Verification items for the finished model (mm, model axes). A direction names the side the tool comes from. Give positions to 0.01 mm unless a question says otherwise; leave off trailing zeros. Loops run counter-clockwise (first coordinate to the right, second up) from the corner with the lowest first, then second, coordinate; pieces in that order, holes last. Notation, with made-up numbers: (-7, 77) - (14, 77) arc R22 cw to (14, 110) - close; hole circle Ø6 at (52, -29.5). An arc over 180 degrees is marked (long way). One line per question, with ' | ' between items. Start each with the question number.
1. Section check A-A, the plane y = 16. Enter the section's corners in (x, z).
2. Section check C-C, the plane y = 3.5. Enter the section's corners in (x, z).
3. Thickness scan on line 1 along X through (y, z) = (16, 15.6); line 2 along Y through (x, z) = (19.75, 14.95); line 3 along X through (y, z) = (-17, 13.25). Record the ranges inside material, lowest first. Write a range as from..to.
4. Section check B-B, the plane z = 10.5. Enter the section's corners in (x, y).
5. Depth check by flat-ended pin: pin 1 Ø3 at (x, z) = (18.5, 8.5) entering from -Y; pin 2 Ø16 at (x, y) = (4, 4.5) entering from +Z; pin 3 Ø5.5 at (y, z) = (-15, 6.5) entering from -X. Enter the tip coordinate at first touch or a pass-through.
6. Mould release check, pull along Y, two halves, no side actions. Record for faces 1 (the face through (-16, 0, 1)), 2 (the face through (-16.792, -18.746, 3.522)), 3 (the face through (-17.4, 19.1, 1.4)): +Y half, -Y half, draft (parallel to the pull), parting line (faces both ways), or undercut.
7. Tool access check on faces 4 (the face through (-17.2, 12.7, 1.8)), 5 (the face through (17, 18.5, 12)), 6 (the face through (-17, -18.5, 12)), 7 (the face through (16, 0, 1)). Record the directions out of +Z, -Z, +X, -X, +Y, -Y that give a thin tool (end or side, any length) a straight path to the whole face; none if there is none.
8. Section check D-D, the plane x = 2.5. Enter the section's corners in (y, z), then the cut area to 3 significant figures.
from build123d import *

# Parameters (mm, degrees)
SKETCH1_W               = 32
SKETCH1_H               = 40
BOSS_EXTRUDE1_DEPTH     = 1.5
SKETCH2_R               = 1.2
BOSS_EXTRUDE2_DEPTH     = 16.5
CUT_EXTRUDE1_DEPTH      = 35.165955277
CUT_EXTRUDE1_DEPTH_BACK = 35.165955277
SKETCH4_W               = 10
SKETCH4_H               = 14.5
CHAMFER1_SIZE           = 2
FILLET1_R               = 5


with BuildPart() as part:
    # Sketch1 → Boss-Extrude1 (new body)
    with BuildSketch(Plane.XY):
        Rectangle(SKETCH1_W, SKETCH1_H)
    extrude(amount=BOSS_EXTRUDE1_DEPTH)

    # Sketch2 → Boss-Extrude2 (add)
    # profile 1 of 4: a face of its own
    with BuildSketch(Plane.XY):
        with BuildLine():
            Line((-16, 18.5), (-19.75, 18.5))
            ThreePointArc((-19.75, 18.5), (-22.25, 16), (-19.75, 13.5))
            Line((-19.75, 13.5), (-16, 13.5))
            Line((-16, 13.5), (-16, 18.5))
        make_face()
        with Locations((-19.75, 16)):
            Circle(SKETCH2_R, mode=Mode.SUBTRACT)
    # profile 2 of 4: a face of its own
    with BuildSketch(Plane.XY):
        with BuildLine():
            Line((16, 18.5), (16, 13.5))
            Line((16, 13.5), (19.75, 13.5))
            ThreePointArc((19.75, 13.5), (22.25, 16), (19.75, 18.5))
            Line((19.75, 18.5), (16, 18.5))
        make_face()
        with Locations(Location((19.75, 16, 0), (0, 0, 180))):
            Circle(SKETCH2_R, mode=Mode.SUBTRACT)
    # profile 3 of 4: a face of its own
    with BuildSketch(Plane.XY):
        with BuildLine():
            Line((16, -18.5), (19.75, -18.5))
            ThreePointArc((19.75, -18.5), (22.25, -16), (19.75, -13.5))
            Line((19.75, -13.5), (16, -13.5))
            Line((16, -13.5), (16, -18.5))
        make_face()
        with Locations((19.75, -16)):
            Circle(SKETCH2_R, mode=Mode.SUBTRACT)
    # profile 4 of 4: a face of its own
    with BuildSketch(Plane.XY):
        with BuildLine():
            Line((-16, -18.5), (-16, -13.5))
            Line((-16, -13.5), (-19.75, -13.5))
            ThreePointArc((-19.75, -13.5), (-22.25, -16), (-19.75, -18.5))
            Line((-19.75, -18.5), (-16, -18.5))
        make_face()
        with Locations(Location((-19.75, -16, 0), (0, 0, 180))):
            Circle(SKETCH2_R, mode=Mode.SUBTRACT)
    extrude(amount=BOSS_EXTRUDE2_DEPTH)

    # Sketch4 → Cut-Extrude1 (cut, two sides: drawn at the far end of the back side and taken through both)
    with BuildSketch(Plane(origin=(0, 0, 0), x_dir=(1, 0, 0), z_dir=(0, 1, 0)).offset(-CUT_EXTRUDE1_DEPTH_BACK)):
        with Locations((-23, -7.25)):
            Rectangle(SKETCH4_W, SKETCH4_H)
        with Locations((23, -7.25)):
            Rectangle(SKETCH4_W, SKETCH4_H)
    extrude(amount=CUT_EXTRUDE1_DEPTH + CUT_EXTRUDE1_DEPTH_BACK, mode=Mode.SUBTRACT)

    # Chamfer1
    # the kernel refuses this chamfer: 2 mm, written as the material it adds along each edge
    with BuildSketch(Plane(origin=(-16, -13.5, 0), x_dir=(-1, 0, 0), z_dir=(0, 0, 1)), Plane(origin=(-16, 13.5, 0), x_dir=(0, -1, 0), z_dir=(0, 0, 1)), Plane(origin=(16, -13.5, 0), x_dir=(0, 1, 0), z_dir=(0, 0, 1)), Plane(origin=(16, 13.5, 0), x_dir=(1, 0, 0), z_dir=(0, 0, 1))) as chamfer1_piece_1:
        Polygon((CHAMFER1_SIZE, 0), (0, -CHAMFER1_SIZE), (0, 0), align=None)
    extrude(amount=1.5)
    with BuildSketch(Plane(origin=(-16, -18.5, 0), x_dir=(0, -1, 0), z_dir=(0, 0, 1))) as chamfer1_piece_2_section:
        Polygon((CHAMFER1_SIZE, 0), (0, -CHAMFER1_SIZE), (0, 0), align=None)
    chamfer1_piece_2 = extrude(amount=1.5, mode=Mode.PRIVATE)
    chamfer1_piece_2 = split(chamfer1_piece_2, bisect_by=Plane(origin=(-16, -20, 0), z_dir=(0, 1, 0)), keep=Keep.TOP, mode=Mode.PRIVATE)
    add(chamfer1_piece_2)
    with BuildSketch(Plane(origin=(-16, 18.5, 0), x_dir=(0, 1, 0), z_dir=(0, 0, 1))) as chamfer1_piece_3_section:
        Polygon((CHAMFER1_SIZE, 0), (0, CHAMFER1_SIZE), (0, 0), align=None)
    chamfer1_piece_3 = extrude(amount=1.5, mode=Mode.PRIVATE)
    chamfer1_piece_3 = split(chamfer1_piece_3, bisect_by=Plane(origin=(-16, 20, 0), z_dir=(0, -1, 0)), keep=Keep.TOP, mode=Mode.PRIVATE)
    add(chamfer1_piece_3)
    with BuildSketch(Plane(origin=(16, -18.5, 0), x_dir=(1, 0, 0), z_dir=(0, 0, 1))) as chamfer1_piece_4_section:
        Polygon((CHAMFER1_SIZE, 0), (0, -CHAMFER1_SIZE), (0, 0), align=None)
    chamfer1_piece_4 = extrude(amount=1.5, mode=Mode.PRIVATE)
    chamfer1_piece_4 = split(chamfer1_piece_4, bisect_by=Plane(origin=(16, -20, 0), z_dir=(0, 1, 0)), keep=Keep.TOP, mode=Mode.PRIVATE)
    add(chamfer1_piece_4)
    with BuildSketch(Plane(origin=(16, 18.5, 0), x_dir=(0, 1, 0), z_dir=(0, 0, 1))) as chamfer1_piece_5_section:
        Polygon((CHAMFER1_SIZE, 0), (0, -CHAMFER1_SIZE), (0, 0), align=None)
    chamfer1_piece_5 = extrude(amount=1.5, mode=Mode.PRIVATE)
    chamfer1_piece_5 = split(chamfer1_piece_5, bisect_by=Plane(origin=(16, 20, 0), z_dir=(0, -1, 0)), keep=Keep.TOP, mode=Mode.PRIVATE)
    add(chamfer1_piece_5)

    # Fillet1
    # the kernel refuses this fillet: 5 mm, written as the material it adds along each edge
    with BuildSketch(Plane(origin=(-16, -13.5, 1.5), x_dir=(0, 0, 1), z_dir=(-1, 0, 0))) as fillet1_piece_1_section:
        with BuildLine():
            CenterArc((FILLET1_R, FILLET1_R), FILLET1_R, 180, 90)
            Line((0, FILLET1_R), (0, 0))
            Line((0, 0), (FILLET1_R, 0))
        make_face()
    fillet1_piece_1 = extrude(amount=14.5, mode=Mode.PRIVATE)
    fillet1_piece_1 = split(fillet1_piece_1, bisect_by=Plane(origin=(-17, -12.5, 1.5), z_dir=(0.7071067811865476, -0.7071067811865476, 0)), keep=Keep.TOP, mode=Mode.PRIVATE)
    add(fillet1_piece_1)
    with BuildSketch(Plane(origin=(-26.926785536, -18.5, 1.5), x_dir=(0, 0, 1), z_dir=(1, 0, 0))) as fillet1_piece_2_section:
        with BuildLine():
            CenterArc((3.570714214, 5), FILLET1_R, 224.427004001, 45.572995999)
            Line((0, 1.5), (0, 0))
            Line((0, 0), (3.570714214, 0))
        make_face()
    fillet1_piece_2 = extrude(amount=10.926785536, mode=Mode.PRIVATE)
    fillet1_piece_2 = split(fillet1_piece_2, bisect_by=Plane(origin=(-22.463392768, -14.036607232, 1.5), z_dir=(0.7071067811865476, 0.7071067811865476, 0)), keep=Keep.TOP, mode=Mode.PRIVATE)
    add(fillet1_piece_2)
    with BuildSketch(Plane(origin=(-30.5, 13.5, 1.5), x_dir=(0, 0, 1), z_dir=(1, 0, 0))) as fillet1_piece_3_section:
        with BuildLine():
            CenterArc((FILLET1_R, FILLET1_R), FILLET1_R, 180, 90)
            Line((0, FILLET1_R), (0, 0))
            Line((0, 0), (FILLET1_R, 0))
        make_face()
    fillet1_piece_3 = extrude(amount=14.5, mode=Mode.PRIVATE)
    fillet1_piece_3 = split(fillet1_piece_3, bisect_by=Plane(origin=(-24.25, 19.75, 1.5), z_dir=(0.7071067811865476, 0.7071067811865476, 0)), keep=Keep.TOP, mode=Mode.PRIVATE)
    add(fillet1_piece_3)
    with BuildSketch(Plane(origin=(-26.926785536, 18.5, 1.5), x_dir=(0, 0, 1), z_dir=(1, 0, 0))) as fillet1_piece_4_section:
        with BuildLine():
            CenterArc((3.570714214, -5), FILLET1_R, 90, 45.572995999)
            Line((0, -1.5), (0, 0))
            Line((0, 0), (3.570714214, 0))
        make_face()
    fillet1_piece_4 = extrude(amount=10.926785536, mode=Mode.PRIVATE)
    fillet1_piece_4 = split(fillet1_piece_4, bisect_by=Plane(origin=(-22.463392768, 14.036607232, 1.5), z_dir=(0.7071067811865476, -0.7071067811865476, 0)), keep=Keep.TOP, mode=Mode.PRIVATE)
    add(fillet1_piece_4)
    with BuildSketch(Plane(origin=(16, -18.5, 1.5), x_dir=(0, 0, 1), z_dir=(1, 0, 0))) as fillet1_piece_5_section:
        with BuildLine():
            CenterArc((3.570714214, 5), FILLET1_R, 224.427004001, 45.572995999)
            Line((0, 1.5), (0, 0))
            Line((0, 0), (3.570714214, 0))
        make_face()
    fillet1_piece_5 = extrude(amount=10.926785536, mode=Mode.PRIVATE)
    fillet1_piece_5 = split(fillet1_piece_5, bisect_by=Plane(origin=(17, -19.5, 1.5), z_dir=(-0.7071067811865476, 0.7071067811865476, 0)), keep=Keep.TOP, mode=Mode.PRIVATE)
    add(fillet1_piece_5)
    with BuildSketch(Plane(origin=(30.5, -13.5, 1.5), x_dir=(0, 0, 1), z_dir=(-1, 0, 0))) as fillet1_piece_6_section:
        with BuildLine():
            CenterArc((FILLET1_R, FILLET1_R), FILLET1_R, 180, 90)
            Line((0, FILLET1_R), (0, 0))
            Line((0, 0), (FILLET1_R, 0))
        make_face()
    fillet1_piece_6 = extrude(amount=14.5, mode=Mode.PRIVATE)
    fillet1_piece_6 = split(fillet1_piece_6, bisect_by=Plane(origin=(24.25, -19.75, 1.5), z_dir=(-0.7071067811865476, -0.7071067811865476, 0)), keep=Keep.TOP, mode=Mode.PRIVATE)
    add(fillet1_piece_6)
    with BuildSketch(Plane(origin=(16, 13.5, 1.5), x_dir=(0, -1, 0), z_dir=(1, 0, 0))) as fillet1_piece_7_section:
        with BuildLine():
            CenterArc((FILLET1_R, -FILLET1_R), FILLET1_R, 90, 90)
            Line((0, -FILLET1_R), (0, 0))
            Line((0, 0), (FILLET1_R, 0))
        make_face()
    fillet1_piece_7 = extrude(amount=14.5, mode=Mode.PRIVATE)
    fillet1_piece_7 = split(fillet1_piece_7, bisect_by=Plane(origin=(17, 12.5, 1.5), z_dir=(-0.7071067811865476, 0.7071067811865476, 0)), keep=Keep.TOP, mode=Mode.PRIVATE)
    add(fillet1_piece_7)
    with BuildSketch(Plane(origin=(26.926785536, 18.5, 1.5), x_dir=(0, 1, 0), z_dir=(-1, 0, 0))) as fillet1_piece_8_section:
        with BuildLine():
            CenterArc((5, -3.570714214), FILLET1_R, 134.427004001, 45.572995999)
            Line((0, -3.570714214), (0, 0))
            Line((0, 0), (1.5, 0))
        make_face()
    fillet1_piece_8 = extrude(amount=10.926785536, mode=Mode.PRIVATE)
    fillet1_piece_8 = split(fillet1_piece_8, bisect_by=Plane(origin=(22.463392768, 14.036607232, 1.5), z_dir=(-0.7071067811865476, -0.7071067811865476, 0)), keep=Keep.TOP, mode=Mode.PRIVATE)
    add(fillet1_piece_8)


solid = part.part
Results list:
1) outline: (-22.25, 14.5) - (-20.95, 14.5) - (-20.95, 16.5) - (-22.25, 16.5) - close; (-18.55, 14.5) - (-18, 14.5) - (-18, 0) - (18, 0) - (18, 14.5) - (18.55, 14.5) - (18.55, 16.5) - (16, 16.5) - (16, 1.5) - (-16, 1.5) - (-16, 16.5) - (-18.55, 16.5) - close; (20.95, 14.5) - (22.25, 14.5) - (22.25, 16.5) - (20.95, 16.5) - close
2) outline: (-16, 0) - (16, 0) - (16, 1.5) - (-16, 1.5) - close
3) line 1: -22.25..-20.95, -18.55..-16, 16..18.55, 20.95..22.25 | line 2: -18.5..-17.2, -14.8..-13.5, 13.5..14.8, 17.2..18.5 | line 3: -18..-16, 16..18
4) outline: (-18, -18.5) - (-16, -18.5) - (-16, -13.5) - (-18, -13.5) - close; (-18, 13.5) - (-16, 13.5) - (-16, 18.5) - (-18, 18.5) - close; (16, -18.5) - (18, -18.5) - (18, -13.5) - (16, -13.5) - close; (16, 13.5) - (18, 13.5) - (18, 18.5) - (16, 18.5) - close
5) pin 1: y = -18.5 | pin 2: z = 1.5 | pin 3: x = -18
6) face 1: undercut | face 2: -Y half | face 3: +Y half
7) face 4: +Z, -Z, -X | face 5: +Z, +X, -X, +Y | face 6: +Z, +X, -X, -Y | face 7: +Z, -Z, +X
8) outline: (-20, 0) - (20, 0) - (20, 1.5) - (-20, 1.5) - close | area: 60.0 mm²
